```python
from build123d import *

# Parameters (mm, degrees)
SKETCH2_R                = 60
SKETCH2_R_2              = 10
BOSS_EXTRUDE1_DEPTH      = 20
SKETCH3_R                = 42.5
CUT_EXTRUDE1_DEPTH       = 10
CUT_EXTRUDE2_START       = -31
SKETCH4_R                = 6
CUT_EXTRUDE2_DEPTH       = 42
CIRPATTERN2_COUNT        = 5
SKETCH6_R                = 13.5
SKETCH6_R_2              = 10
BOSS_EXTRUDE3_DEPTH      = 2
BOSS_EXTRUDE3_DEPTH_BACK = 7
SKETCH8_W                = 6
SKETCH8_H                = 3.21
CUT_EXTRUDE3_DEPTH       = 11
CUT_EXTRUDE3_DEPTH_BACK  = 31


with BuildPart() as part:
    # Sketch2 → Boss-Extrude1 (new body, symmetric)
    with BuildSketch(Plane.XY):
        Circle(SKETCH2_R)
        Circle(SKETCH2_R_2, mode=Mode.SUBTRACT)
    extrude(amount=BOSS_EXTRUDE1_DEPTH, both=True)

    # Sketch3 → Cut-Extrude1 (cut)
    with BuildSketch(Plane.XY.offset(20)):
        Circle(SKETCH3_R)
    cut_extrude1 = extrude(amount=-CUT_EXTRUDE1_DEPTH, mode=Mode.SUBTRACT)

    # Mirror2: Cut-Extrude1 across plane
    add(cut_extrude1.mirror(Plane.XY), mode=Mode.SUBTRACT)

    # Sketch4 → Cut-Extrude2 (cut)
    with BuildSketch(Plane.XY.offset(10).offset(CUT_EXTRUDE2_START)):
        with Locations((0, 25)):
            Circle(SKETCH4_R)
    cut_extrude2 = extrude(amount=CUT_EXTRUDE2_DEPTH, mode=Mode.SUBTRACT)

    # CirPattern2: Cut-Extrude2 ×5 about axis
    cirpattern2_axis = Axis((0, 0, 0), (0, 0, 1))
    for i in range(1, CIRPATTERN2_COUNT):
        add(cut_extrude2.rotate(cirpattern2_axis, i * 360 / CIRPATTERN2_COUNT), mode=Mode.SUBTRACT)

    # Sketch5 → Cut-Revolve1 (revolve, cut)
    with BuildSketch(Plane(origin=(0, 0, 0), x_dir=(1, 0, 0), z_dir=(0, 1, 0))):
        Polygon((54, 13.535898385), (60, 17), (60, -17), (54, -13.535898385), align=None)
    revolve(axis=Axis((0, 0, 0), (0, 0, -1)), mode=Mode.SUBTRACT)

    # Sketch6 → Boss-Extrude3 (add, two sides)
    with BuildSketch(Plane.XY.offset(10)) as boss_extrude3_sk:
        Circle(SKETCH6_R)
        Circle(SKETCH6_R_2, mode=Mode.SUBTRACT)
    extrude(amount=BOSS_EXTRUDE3_DEPTH)
    extrude(boss_extrude3_sk.sketch, amount=-BOSS_EXTRUDE3_DEPTH_BACK)

    # Sketch8 → Cut-Extrude3 (cut, two sides)
    with BuildSketch(Plane(origin=(0, 0, -10), x_dir=(-1, 0, 0), z_dir=(0, 0, -1))) as cut_extrude3_sk:
        with Locations((0, 11.121882551)):
            Rectangle(SKETCH8_W, SKETCH8_H)
    extrude(amount=CUT_EXTRUDE3_DEPTH, mode=Mode.SUBTRACT)
    extrude(cut_extrude3_sk.sketch, amount=-CUT_EXTRUDE3_DEPTH_BACK, mode=Mode.SUBTRACT)


solid = part.part
```
Geometry check sheet. Reference: the model listing, model coordinates, mm. A direction names the side the tool comes from. Coordinates: 2 decimals unless noted, no trailing zeros. Order: outer loops, then holes, each group sorted by start corner. A loop starts at its lowest first (then second) coordinate and runs counter-clockwise, first axis right, second up.
Item 1: Section check A-A (y = 0). Enter the section's corners in (x, z), plus the area to 3 significant figures.
Item 2: Scan lines: line 1 along X through (y, z) = (0, -0.25); line 2 along Y through (x, z) = (-1.5, 11); line 3 along Y through (x, z) = (-1.5, 7). Record each from-to range of solid material in increasing order.
Item 3: Depth check by flat-ended pin: pin 1 (8 mm diameter, centred on x = 36, z = -15.5, fed in from -Y); pin 2 (15.5 mm diameter, centred on x = -14.69, y = -20.23, fed in from +Z); pin 3 (12 mm diameter, centred on x = 40.5, z = 10, fed in from +Y). Enter the tip coordinate at first touch or a pass-through.
Item 4: Section check B-B (z = -8). Enter the section's corners in (x, y).
Item 5: Tool access check on faces 4 (the cylindrical face through (-2.93, -13.18, 10.99)), 5 (the flat face through (3, 11, 1)), 6 (the flat face through (9, -9, -10)). Record the directions out of +Z, -Z, +X, -X, +Y, -Y that give a thin tool (end or side, any length) a straight path to the whole face; none if there is none.
Item 6: Mould release check, pull along X, two halves, no side actions. Record for faces 1 (the cylindrical face through (-59.94, 2.64, -18.48)), 2 (the flat face through (12, 41, 20)), 3 (the cylindrical face through (-27.59, 12.36, -0.14)): released by +X, released by -X, zero draft, split by the parting line, or undercut.
Check sheet entries:
1. outline: (-60, -20) - (-42.5, -20) - (-42.5, -10) - (-10, -10) - (-10, 12) - (-13.5, 12) - (-13.5, 10) - (-42.5, 10) - (-42.5, 20) - (-60, 20) - (-60, 17) - (-54, 13.54) - (-54, -13.54) - (-60, -17) - close; (10, -10) - (42.5, -10) - (42.5, -20) - (60, -20) - (60, -17) - (54, -13.54) - (54, 13.54) - (60, 17) - (60, 20) - (42.5, 20) - (42.5, 10) - (13.5, 10) - (13.5, 12) - (10, 12) - close
1. area: 2,350 mm2
2. line 1: x = -54 to -10, 10 to 54
2. line 2: y = -53.98 to -42.47, -13.42 to -9.89, 12.73 to 13.42, 42.47 to 53.98
2. line 3: y = -53.98 to -9.89, 12.73 to 19.19, 30.81 to 53.98
3. pin 1: stops at y = -50.57
3. pin 2: stops at z = 10
3. pin 3: stops at y = 42.95
4. outline: circle Ø108 at (0, 0); hole circle Ø12 at (-23.78, 7.73); hole circle Ø12 at (-14.69, -20.23); hole circle Ø12 at (0, 25); hole (-3, 9.54) arc R10 ccw (long way) to (3, 9.54) - (3, 12.73) - (-3, 12.73) - close; hole circle Ø12 at (14.69, -20.23); hole circle Ø12 at (23.78, 7.73)
5. face 4: +Z
5. face 5: +Z, -Z
5. face 6: -Z
6. face 1: split by the parting line
6. face 2: zero draft
6. face 3: undercut
